from build123d import *

# Parameters (mm, degrees)
CUT_EXTRUDE1_DEPTH = 8.366
FILLET1_R          = 5
FILLET2_R          = 5
FILLET3_R          = 5
FILLET4_R          = 5
FILLET5_R          = 5
FILLET6_R          = 5
FILLET7_R          = 5
FILLET8_R          = 5
FILLET9_R          = 5
FILLET10_R         = 5
FILLET11_R         = 3
FILLET12_R         = 3
FILLET13_R         = 3
FILLET14_R         = 3
FILLET15_R         = 3
FILLET16_R         = 3
FILLET17_R         = 3
FILLET18_R         = 3
FILLET19_R         = 3
FILLET20_R         = 3
SKETCH4_R          = 2.667
CUT_EXTRUDE2_DEPTH = 8.366


with BuildPart() as part:
    # Sketch1 → Revolve1 (revolve)
    with BuildSketch(Plane.XY):
        with BuildLine():
            Line((1.905, 50.8), (3.683, 50.8))
            Line((3.683, 50.8), (3.683, 0))
            Line((3.683, 0), (-3.683, 0))
            Line((-3.683, 0), (-3.683, 50.8))
            Line((-3.683, 50.8), (-1.905, 50.8))
            ThreePointArc((-1.905, 50.8), (0, 48.895), (1.905, 50.8))
        make_face()
    revolve(axis=Axis((3.683, 0, 0), (-1, 0, 0)))

    # Sketch2 → Cut-Extrude1 (cut, through all)
    with BuildSketch(Plane(origin=(3.683, 0, 0), x_dir=(0, 0, -1), z_dir=(1, 0, 0))):
        with BuildLine():
            Line((-5.367251924, 11.510108895), (-17.175206157, 36.832348465))
            ThreePointArc((-17.175206157, 36.832348465), (0, 40.64), (17.175206157, 36.832348465))
            Line((17.175206157, 36.832348465), (5.367251924, 11.510108895))
            ThreePointArc((5.367251924, 11.510108895), (0, 12.7), (-5.367251924, 11.510108895))
        make_face()
        with BuildLine():
            Line((9.288192011, 8.661379173), (29.722214434, 27.716413353))
            ThreePointArc((29.722214434, 27.716413353), (38.650936822, 12.558450651), (40.337075603, -4.952770116))
            Line((40.337075603, -4.952770116), (12.605336126, -1.547740661))
            ThreePointArc((12.605336126, -1.547740661), (12.078417757, 3.924515829), (9.288192011, 8.661379173))
        make_face()
        with BuildLine():
            Line((11.107670281, -6.157082177), (35.544544898, -19.702662967))
            ThreePointArc((35.544544898, -19.702662967), (23.887592653, -32.878450651), (7.754477572, -39.893328735))
            Line((7.754477572, -39.893328735), (2.423274241, -12.46666523))
            ThreePointArc((2.423274241, -12.46666523), (7.464872704, -10.274515829), (11.107670281, -6.157082177))
        make_face()
        with BuildLine():
            Line((-2.423274241, -12.46666523), (-7.754477572, -39.893328735))
            ThreePointArc((-7.754477572, -39.893328735), (-23.887592653, -32.878450651), (-35.544544898, -19.702662967))
            Line((-35.544544898, -19.702662967), (-11.107670281, -6.157082177))
            ThreePointArc((-11.107670281, -6.157082177), (-7.464872704, -10.274515829), (-2.423274241, -12.46666523))
        make_face()
        with BuildLine():
            Line((-12.605336126, -1.547740661), (-40.337075603, -4.952770116))
            ThreePointArc((-40.337075603, -4.952770116), (-38.650936822, 12.558450651), (-29.722214434, 27.716413353))
            Line((-29.722214434, 27.716413353), (-9.288192011, 8.661379173))
            ThreePointArc((-9.288192011, 8.661379173), (-12.078417757, 3.924515829), (-12.605336126, -1.547740661))
        make_face()
    extrude(amount=-CUT_EXTRUDE1_DEPTH, mode=Mode.SUBTRACT)

    # Fillet1
    fillet1_edges = [part.edges().sort_by_distance(p)[0] for p in [
        (0, -39.893328735, -7.754477572),
    ]]
    fillet(fillet1_edges, radius=FILLET1_R)

    # Fillet2
    fillet2_edges = [part.edges().sort_by_distance(p)[0] for p in [
        (0, -19.702662967, -35.544544898),
    ]]
    fillet(fillet2_edges, radius=FILLET2_R)

    # Fillet3
    fillet3_edges = [part.edges().sort_by_distance(p)[0] for p in [
        (0, 27.716413353, -29.722214434),
    ]]
    fillet(fillet3_edges, radius=FILLET3_R)

    # Fillet4
    fillet4_edges = [part.edges().sort_by_distance(p)[0] for p in [
        (0, -4.952770116, -40.337075603),
    ]]
    fillet(fillet4_edges, radius=FILLET4_R)

    # Fillet5
    fillet5_edges = [part.edges().sort_by_distance(p)[0] for p in [
        (0, 36.832348465, -17.175206157),
    ]]
    fillet(fillet5_edges, radius=FILLET5_R)

    # Fillet6
    fillet6_edges = [part.edges().sort_by_distance(p)[0] for p in [
        (0, 36.832348465, 17.175206157),
    ]]
    fillet(fillet6_edges, radius=FILLET6_R)

    # Fillet7
    fillet7_edges = [part.edges().sort_by_distance(p)[0] for p in [
        (0, -4.952770116, 40.337075603),
    ]]
    fillet(fillet7_edges, radius=FILLET7_R)

    # Fillet8
    fillet8_edges = [part.edges().sort_by_distance(p)[0] for p in [
        (0, 27.716413353, 29.722214434),
    ]]
    fillet(fillet8_edges, radius=FILLET8_R)

    # Fillet9
    fillet9_edges = [part.edges().sort_by_distance(p)[0] for p in [
        (0, -19.702662967, 35.544544898),
    ]]
    fillet(fillet9_edges, radius=FILLET9_R)

    # Fillet10
    fillet10_edges = [part.edges().sort_by_distance(p)[0] for p in [
        (0, -39.893328735, 7.754477572),
    ]]
    fillet(fillet10_edges, radius=FILLET10_R)

    # Fillet11
    fillet11_edges = [part.edges().sort_by_distance(p)[0] for p in [
        (0, 11.510108895, 5.367251924),
    ]]
    fillet(fillet11_edges, radius=FILLET11_R)

    # Fillet12
    fillet12_edges = [part.edges().sort_by_distance(p)[0] for p in [
        (0, 11.510108895, -5.367251924),
    ]]
    fillet(fillet12_edges, radius=FILLET12_R)

    # Fillet13
    fillet13_edges = [part.edges().sort_by_distance(p)[0] for p in [
        (0, -1.547740661, 12.605336126),
    ]]
    fillet(fillet13_edges, radius=FILLET13_R)

    # Fillet14
    fillet14_edges = [part.edges().sort_by_distance(p)[0] for p in [
        (0, 8.661379173, 9.288192011),
    ]]
    fillet(fillet14_edges, radius=FILLET14_R)

    # Fillet15
    fillet15_edges = [part.edges().sort_by_distance(p)[0] for p in [
        (0, -6.157082177, 11.107670281),
    ]]
    fillet(fillet15_edges, radius=FILLET15_R)

    # Fillet16
    fillet16_edges = [part.edges().sort_by_distance(p)[0] for p in [
        (0, -12.46666523, 2.423274241),
    ]]
    fillet(fillet16_edges, radius=FILLET16_R)

    # Fillet17
    fillet17_edges = [part.edges().sort_by_distance(p)[0] for p in [
        (0, -12.46666523, -2.423274241),
    ]]
    fillet(fillet17_edges, radius=FILLET17_R)

    # Fillet18
    fillet18_edges = [part.edges().sort_by_distance(p)[0] for p in [
        (0, -6.157082177, -11.107670281),
    ]]
    fillet(fillet18_edges, radius=FILLET18_R)

    # Fillet19
    fillet19_edges = [part.edges().sort_by_distance(p)[0] for p in [
        (0, -1.547740661, -12.605336126),
    ]]
    fillet(fillet19_edges, radius=FILLET19_R)

    # Fillet20
    fillet20_edges = [part.edges().sort_by_distance(p)[0] for p in [
        (0, 8.661379173, -9.288192011),
    ]]
    fillet(fillet20_edges, radius=FILLET20_R)

    # Sketch4 → Cut-Extrude2 (cut, through all)
    with BuildSketch(Plane.ZY.offset(3.683)):
        Circle(SKETCH4_R)
    extrude(amount=-CUT_EXTRUDE2_DEPTH, mode=Mode.SUBTRACT)


solid = part.part
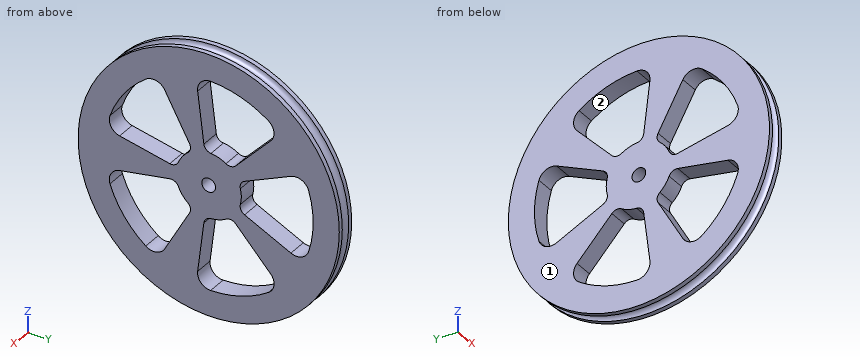
Could you check a few things on this model? Use its own coordinates, in mm. Face numbers are marked on the shaded views. Coordinates: 2 decimals unless noted, no trailing zeros. Order: outer loops, then holes, each group sorted by start corner. A loop starts at its lowest first (then second) coordinate and runs counter-clockwise, first axis right, second up. Notation, with made-up numbers: (54, -26.5) - (90, -26.5) arc R23 ccw to (90, -8.5) - close; hole circle Ø7 at (83.5, -8). An arc over 180 degrees is marked (long way). Answer in a Markdown table with one row per item. Add a question column.
(1) I need wall thicknesses on L1, parallel to Y at x = 2, z = 0; L2, parallel to Z at x = 3, y = 21; L3, parallel to Z at x = -0.5, y = 5.5. Which ranges of each line are inside material? Lowest first, please.
(2) If we mould it in two halves opening along Y, with no side actions, what happens to the marked faces 1 and 2? For each: released by +Y, released by -Y, zero draft, split by the parting line, or undercut.
(3) Will these pins go through, and if not, where does the flat tip stop? pin 1 (3 mm diameter, centred on x = 0, z = 27.5, fed in from -Y); pin 2 (12 mm diameter, centred on y = -31.5, z = -14, fed in from -X); pin 3 (2 mm diameter, centred on x = -1, z = -13.5, fed in from -Y).
(4) If we section it at A-A, the plane z = 0: Please give me the cut outline in (x, y) (3 decimals).
(5) If we section it at B-B, the plane y = -36: State how many separate pieces and enclosed holes the cut face has, then the cut area to 3 significant figures.
Results are:
| question | item | result |
|---|---|---|
| 1 | L1 | y = -50.8 to -2.67, 2.67 to 12.7, 40.64 to 50.8 |
| 1 | L2 | z = -46.26 to -34.79, -22.52 to -9.79, 9.79 to 22.52, 34.79 to 46.26 |
| 1 | L3 | z = -48.65 to -40.27, -11.45 to 11.45, 40.27 to 48.65 |
| 2 | face 1 | zero draft |
| 2 | face 2 | undercut |
| 3 | pin 1 | stops at y = -41.54 |
| 3 | pin 2 | passes through |
| 3 | pin 3 | stops at y = -49.09 |
| 4 | outline | (-3.683, -50.8) - (-1.905, -50.8) arc R1.905 cw to (1.905, -50.8) - (3.683, -50.8) - (3.683, -2.667) - (-3.683, -2.667) - close; (-3.683, 2.667) - (3.683, 2.667) - (3.683, 12.7) - (-3.683, 12.7) - close; (-3.683, 40.64) - (3.683, 40.64) - (3.683, 50.8) - (1.905, 50.8) arc R1.905 cw to (-1.905, 50.8) - (-3.683, 50.8) - close |
| 5 | separate pieces | 3 |
| 5 | enclosed holes | 0 |
| 5 | area | 340 mm2 |
